from build123d import *

# Parameters (mm, degrees)
SKETCH1_W              = 58
SKETCH1_H              = 40
BOSS_EXTRUDE1_DEPTH    = 6
BOSS_EXTRUDE3_START    = -2.6
BOSS_EXTRUDE3_DEPTH    = 42
SKETCH6_W              = 6
SKETCH6_H              = 7.4
BOSS_EXTRUDE4_DEPTH    = 20
BOSS_EXTRUDE5_DEPTH    = 10
M2_5_CLEARANCE_SLOT1_D = 2.9
SKETCH11_R             = 1.75
CUT_EXTRUDE1_DEPTH     = 10
SKETCH12_W             = 8
SKETCH12_H             = 40
SKETCH12_R             = 1.65
BOSS_EXTRUDE6_DEPTH    = 3
FILLET1_R              = 2
SKETCH8_R              = 3.9
CUT_EXTRUDE2_DEPTH     = 5


with BuildPart() as part:
    # Sketch1 → Boss-Extrude1 (new body)
    with BuildSketch(Plane(origin=(0, 0, 0), x_dir=(1, 0, 0), z_dir=(0, 1, 0))):
        Rectangle(SKETCH1_W, SKETCH1_H)
    extrude(amount=BOSS_EXTRUDE1_DEPTH)

    # Sketch4 → Boss-Extrude3 (add)
    with BuildSketch(Plane.ZY.offset(29).offset(BOSS_EXTRUDE3_START)):
        Polygon((-20, 6), (19.918609503, 43.543902506), (20, 6), align=None)
    extrude(amount=-BOSS_EXTRUDE3_DEPTH)

    # Sketch6 → Boss-Extrude4 (add)
    with BuildSketch(Plane(origin=(0, 13.164986139, -12.38181796), x_dir=(1, 0, 0), z_dir=(0, 0.728441779, -0.68510771))):
        with Locations((-10.9, -40.641810675)):
            Rectangle(SKETCH6_W, SKETCH6_H)
        with Locations((-10.9, 6.758189325)):
            Rectangle(SKETCH6_W, SKETCH6_H)
    extrude(amount=BOSS_EXTRUDE4_DEPTH)

    # Sketch7 → Boss-Extrude5 (add)
    with BuildSketch(Plane(origin=(29, 0, 0), x_dir=(0, 0, -1), z_dir=(1, 0, 0))):
        with BuildLine():
            Line((-20, 6), (-13.364634961, 10.800412746))
            ThreePointArc((-13.364634961, 10.800412746), (-8.798657798, 16.130102837), (-7.156866334, 22.953464523))
            Line((-7.156866334, 22.953464523), (-7.156866334, 39.25))
            ThreePointArc((-7.156866334, 39.25), (-0.756866334, 45.65), (5.643133666, 39.25))
            Line((5.643133666, 39.25), (5.643133666, 22.953464523))
            ThreePointArc((5.643133666, 22.953464523), (7.651002835, 15.456496038), (13.137071863, 9.966585137))
            Line((13.137071863, 9.966585137), (20, 6))
            Line((20, 6), (-20, 6))
        make_face()
    extrude(amount=-BOSS_EXTRUDE5_DEPTH)

    # M2.5 Clearance Slot1 (through all)
    with Locations(Plane(origin=(-16.9, -75.052586312, -128.704072023), x_dir=(0, -0.380749805, 0.924678098), z_dir=(-1, 0, 0))):
        with Locations((57.189532403, 125.168887287), (66.298114004, 121.041691966), (77.412789478, 169.800937131), (86.521371079, 165.67374181)):
            Hole(M2_5_CLEARANCE_SLOT1_D / 2)

    # Sketch11 → Cut-Extrude1 (cut)
    with BuildSketch(Plane(origin=(29, 0, 0), x_dir=(0, 0, -1), z_dir=(1, 0, 0))):
        with Locations((-0.756866334, 39.25)):
            Circle(SKETCH11_R)
    extrude(amount=-CUT_EXTRUDE1_DEPTH, mode=Mode.SUBTRACT)

    # Sketch12 → Boss-Extrude6 (add)
    with BuildSketch(Plane(origin=(0, 0, 0), x_dir=(1, 0, 0), z_dir=(0, 1, 0))):
        with Locations((33, 0)):
            Rectangle(SKETCH12_W, SKETCH12_H)
        with Locations((33, -15)):
            Circle(SKETCH12_R, mode=Mode.SUBTRACT)
        with Locations((33, 15)):
            Circle(SKETCH12_R, mode=Mode.SUBTRACT)
        with Locations((-33, 0)):
            Rectangle(SKETCH12_W, SKETCH12_H)
        with Locations((-33, 15)):
            Circle(SKETCH12_R, mode=Mode.SUBTRACT)
        with Locations((-33, -15)):
            Circle(SKETCH12_R, mode=Mode.SUBTRACT)
    extrude(amount=BOSS_EXTRUDE6_DEPTH)

    # Fillet1
    fillet1_edges = [part.edges().sort_by_distance(p)[0] for p in [
        (29, 3, 0),
        (-29, 3, 0),
    ]]
    fillet(fillet1_edges, radius=FILLET1_R)

    # Sketch8 → Cut-Extrude2 (cut)
    with BuildSketch(Plane(origin=(29, 0, 0), x_dir=(0, 0, -1), z_dir=(1, 0, 0))):
        with Locations((-0.756866334, 39.25)):
            Circle(SKETCH8_R)
    extrude(amount=-CUT_EXTRUDE2_DEPTH, mode=Mode.SUBTRACT)


solid = part.part
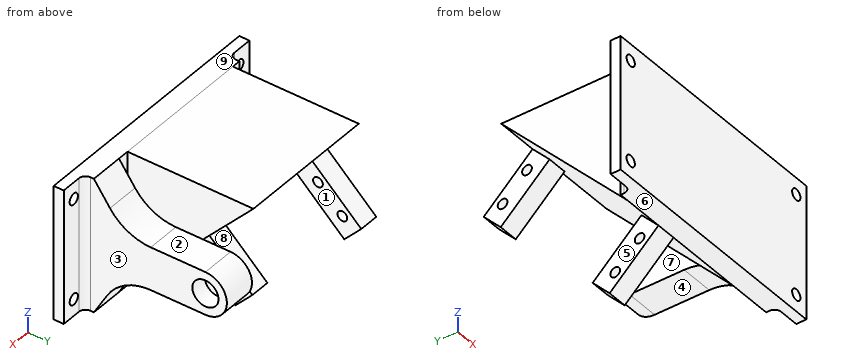
Geometry check sheet. Reference: the model listing, model coordinates, mm. Face numbers are marked on the shaded views. A direction names the side the tool comes from. Round coordinates to 2 decimals unless told otherwise and drop trailing zeros. Order: outer loops, then holes, each group sorted by start corner. A loop starts at its lowest first (then second) coordinate and runs counter-clockwise, first axis right, second up. Notation, with made-up numbers: (48, -10) -> (91, -10) arc R20 ccw to (91, 0) -> close; hole circle Ø4 at (25, 11). An arc over 180 degrees is marked (long way). Use one line per item in the form item = value.
1. Cross-section at C-C, the plane x = 11. Enter the section's corners in (y, z), plus the area to 3 significant figures.
Working result:
outline = (0, -20) -> (6, -20) -> (43.54, 19.92) -> (6, 20) -> (0, 20) -> close
area = 991 mm^2
2. Cross-section at A-A, the plane x = -33. Enter the section's corners in (y, z), plus the area to 3 significant figures.
Working result:
outline = (0, -20) -> (3, -20) -> (3, -16.65) -> (0, -16.65) -> close; (0, -13.35) -> (3, -13.35) -> (3, 13.35) -> (0, 13.35) -> close; (0, 16.65) -> (3, 16.65) -> (3, 20) -> (0, 20) -> close
area = 100 mm^2
3. Go/stop test with flat-tipped pins: pin 1 (2 mm diameter, centred on x = 16.5, z = 4, fed in from -Y); pin 2 (8 mm diameter, centred on x = 9, y = 27.5, fed in from +Z); pin 3 (1.8 mm diameter, centred on x = 3, y = 3, fed in from -Z); pin 4 (15.5 mm diameter, centred on y = 45, z = 9, fed in from +X). Record where each tip stops, or that it passes through.
Working result:
pin_1 = 0
pin_2 = 19.96
pin_3 = -20
pin_4 = 29
4. Set-up check for the marked faces 1, 2, 3, 4 and 5: record each of +Z, -Z, +X, -X, +Y, -Y from which the full face is reachable in a straight line by a thin tool's end or side.
Working result:
face_1 = -Z, +X, +Y
face_2 = +Z, +X, +Y
face_3 = +Z, -Z, +X, +Y
face_4 = -Z, +X, -X, +Y
face_5 = -Z, -X, +Y
5. Mould release check, pull along Z, two halves, no side actions. Record for the marked faces 6, 7, 8 and 9: pulls with the +Z half, pulls with the -Z half, needs draft (parallel to the pull), parting line crosses it, or undercut.
Working result:
face_6 = pulls with the -Z half
face_7 = needs draft
face_8 = undercut
face_9 = pulls with the +Z half
6. Cross-section at B-B, the plane y = 16.5. Enter the section's corners in (x, z), plus the area to 3 significant figures.
Working result:
outline = (-26.4, -8.84) -> (15.6, -8.84) -> (15.6, 19.98) -> (-26.4, 19.98) -> close; (-13.9, -29.88) -> (-7.9, -29.88) -> (-7.9, -19.72) -> (-13.9, -19.72) -> close; (19, -7.1) -> (29, -7.1) -> (29, 8.62) -> (19, 8.62) -> close
area = 1,430 mm^2
7. Scan lines: line 1 along X through (y, z) = (0.75, -15); line 2 along Z through (x, y) = (33, 0.8); line 3 along Z through (x, y) = (-9, 18.5). Record each from-to range of solid material in increasing order. Write a range as from..to.
Working result:
line_1 = -37..-34.65, -31.35..31.35, 34.65..37
line_2 = -20..-16.65, -13.35..13.35, 16.65..20
line_3 = -31.76..-29.55, -26.77..-21.6, -6.71..19.97
